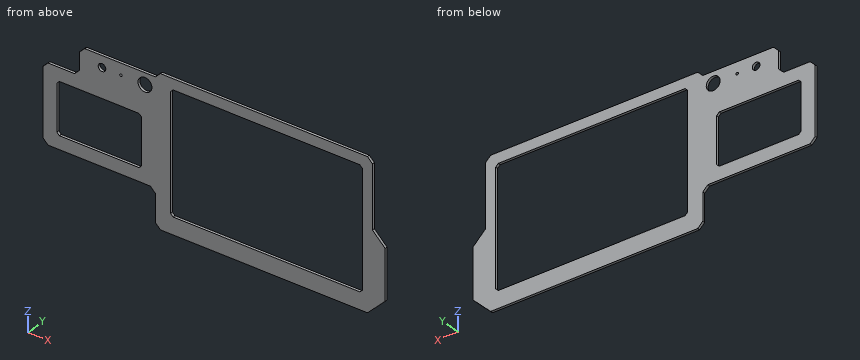
Autodesk Inventor part; units mm, degrees
ref_plane "YZ Plane" through (0, 0, 0) normal (1, 0, 0) x (0, 1, 0)
ref_plane "XZ Plane" through (0, 0, 0) normal (0, 1, 0) x (-1, 0, 0)
ref_plane "XY Plane" through (0, 0, 0) normal (0, 0, 1) x (1, 0, 0)
sketch "Sketch1" plane through (0, 0, 0) normal (0, 1, 0) x (-1, 0, 0)
  line L0 (0, -41) -> (-67, -41)
  line L1 (-67, -41) -> (-67, 0)
  line L2 (-67, 0) -> (0, 0)
  line L3 (0, 0) -> (0, -41)
  line L4 (-90, -68) -> (-242, -68)
  line L5 (-242, -68) -> (-242, 28)
  line L6 (-242, 28) -> (-90, 28)
  line L7 (-90, 28) -> (-90, -68)
  line L8 (11, -47.5) -> (11, 6.5)
  line L9 (7, 10.5) -> (-74, 10.5)
  line L10 (-78, 14.5) -> (-78, 32.5)
  line L11 (-82, 36.5) -> (-246, 36.5)
  line L12 (-250, 32.5) -> (-250, -77.5)
  line L13 (-246, -81.5) -> (-82, -81.5)
  line L14 (-78, -77.5) -> (-78, -55.5)
  line L15 (-74, -51.5) -> (7, -51.5)
  line L16 (11, -47.5) -> (7, -51.5)
  line L17 (-74, -51.5) -> (-78, -55.5)
  line L18 (-78, -77.5) -> (-82, -81.5)
  line L19 (-246, -81.5) -> (-250, -77.5)
  line L20 (-250, 32.5) -> (-246, 36.5)
  line L21 (-82, 36.5) -> (-78, 32.5)
  line L22 (-78, 14.5) -> (-74, 10.5)
  line L23 (7, 10.5) -> (11, 6.5)
  line L24 (6, -46.5) -> (-73, -46.5) construction
  line L25 (-73, -46.5) -> (-73, 5.5) construction
  line L26 (-73, 5.5) -> (6, 5.5) construction
  line L27 (6, 5.5) -> (6, -46.5) construction
  line L28 (-83, -76.5) -> (-245, -76.5) construction
  line L29 (-245, -76.5) -> (-245, 31.5) construction
  line L30 (-245, 31.5) -> (-83, 31.5) construction
  line L31 (-83, 31.5) -> (-83, -76.5) construction
  point P0 (11, 10.5)
  point P1 (-78, 10.5)
  point P2 (-78, 36.5)
  point P3 (-250, 36.5)
  point P4 (-250, -81.5)
  point P5 (-78, -81.5)
  point P6 (-78, -51.5)
  point P7 (11, -51.5)
  point P8 (-33.5, -46.5)
  point P9 (-33.5, -41)
  point P10 (6, -20.5)
  point P11 (0, -20.5)
  point P12 (-83, -22.5)
  point P13 (-90, -20)
  point P14 (-164, -76.5)
  point P15 (-166, -68)
  dimension "d0" = 67
  dimension "d1" = 41
  dimension "d2" = 152
  dimension "d3" = 96
  dimension "d4" = 4
  dimension "d5" = 4
  dimension "d6" = 4
  dimension "d7" = 4
  dimension "d8" = 4
  dimension "d9" = 4
  dimension "d10" = 4
  dimension "d11" = 4
  dimension "d12" = 4
  dimension "d13" = 4
  dimension "d14" = 4
  dimension "d15" = 4
  dimension "d16" = 4
  dimension "d17" = 4
  dimension "d18" = 4
  dimension "d19" = 4
  dimension "d20" = 79
  dimension "d21" = 52
  dimension "d22" = 162
  dimension "d23" = 108
  dimension "d24" = 10
  dimension "d25" = 26
  dimension "d26" = 5
  dimension "d27" = 5
  dimension "d28" = 5
  dimension "d29" = 5
  dimension "d30" = 5
  dimension "d31" = 5
  dimension "d32" = 5
  dimension "d48" = 8.5
  dimension "d49" = 7
extrude "Extrusion1" add sketch "Sketch1" along normal blind 2
sketch "Sketch2" plane through (0, 2, 0) normal (0, 1, 0) x (1, 0, 0)
  line L0 (250, -32.5) -> (250, 77.5)
  line L1 (78, 55.5) -> (74, 51.5)
  line L2 (74, 51.5) -> (-7, 51.5)
  line L3 (250, 77.5) -> (260, 67.5)
  line L4 (260, 67.5) -> (260, 27.5)
  line L5 (260, 27.5) -> (250, 17.5)
  line L6 (250, 77.5) -> (250, 17.5)
  dimension "d35" = 10
  dimension "d36" = 40
extrude "Extrusion2" add sketch "Sketch2" against normal blind 2
sketch "Sketch3" plane through (0, 2, 0) normal (0, 1, 0) x (1, 0, 0)
  line L0 (-7, -10.5) -> (74, -10.5)
  line L1 (74, -10.5) -> (78, -14.5)
  line L2 (78, -14.5) -> (78, -32.5)
  line L3 (78, 55.5) -> (74, 51.5)
  line L4 (74, 51.5) -> (-7, 51.5)
  line L5 (78, -32.5) -> (22, -32.5)
  line L6 (18, -28.5) -> (18, -14.5)
  line L7 (18, -14.5) -> (14, -10.5)
  line L8 (18, -28.5) -> (22, -32.5)
  line L9 (14, -10.5) -> (74, -10.5)
  line L10 (74, -10.5) -> (78, -14.5)
  line L11 (78, -14.5) -> (78, -32.5)
  point P0 (18, -32.5)
  dimension "d39" = 4
  dimension "d40" = 4
  dimension "d41" = 4
  dimension "d42" = 60
extrude "Extrusion3" add sketch "Sketch3" against normal blind 2
chamfer "Chamfer1" distance 2 angle 45 8 edges at (0, 1, -41) (67, 1, -41) (90, 1, -68) (90, 1, 28) (0, 1, 0) (67, 1, 0) (242, 1, 28) (242, 1, -68)
sketch "Sketch4" plane through (0, 2, 0) normal (0, 1, 0) x (1, 0, 0)
  line L0 (18, -14.5) -> (18, -28.5)
  line L1 (22, -32.5) -> (78, -32.5)
  circle A0 centre (69.75, -23.4) radius 5.5
  circle A1 centre (50.75, -23.4) radius 1
  circle A2 centre (35.75, -23.4) radius 3
  point P0 (0, 0)
  dimension "d50" = 11
  dimension "d51" = 2
  dimension "d52" = 6
  dimension "d53" = 19
  dimension "d54" = 15
  dimension "d55" = 9.1
  dimension "d56" = 51.75
extrude "Extrusion4" cut sketch "Sketch4" against normal through all
equation "\"d26\" = 0.5 * d24"
equation "\"d27\" = d26"
equation "\"d28\" = d27"
equation "\"d29\" = d28"
equation "\"d30\" = d26"
equation "\"d31\" = d30"
equation "\"d32\" = d30"
properties part number "front_panel_frame" material "ABS Plastic"
Verification items for the finished model (mm, model axes). Coordinates: 2 decimals unless noted, no trailing zeros. Loops run counter-clockwise (first coordinate to the right, second up) from the corner with the lowest first, then second, coordinate; pieces in that order, holes last. Notation, with made-up numbers: (36, 44) -> (85, 44) arc R11 cw to (85, 56) -> close; hole circle Ø1 at (48.5, 27.5). An arc over 180 degrees is marked (long way). Answer as a JSON object with one key per item and string values. Group by question number.
Item 1: Sectioned sample at B-B on x = 211. Record the boundary of the cut face in (y, z).
Item 2: Scan lines: probe 1 along Z at (x, y) = (50.75, 0.85); probe 2 along Z at (x, y) = (35.75, 0.65); probe 3 along X at (y, z) = (0.25, -17). Record each from-to range of solid material in increasing order.
Item 3: Depth check by flat-ended pin: pin 1 (1 mm diameter, centred on y = 0.5, z = 22.5, fed in from -X); pin 2 (2.5 mm diameter, centred on x = 50.75, z = 23.4, fed in from -Y); pin 3 (1 mm diameter, centred on x = 44.5, y = 1, fed in from +Z); pin 4 (1 mm diameter, centred on x = 19.5, y = 1, fed in from +Z). Enter the tip coordinate at first touch or a pass-through.
Item 4: Sectioned sample at C-C on x = 69.75. Record the boundary of the cut face in (y, z).
Item 5: Sectioned sample at D-D on y = 1.5. State how many separate pieces and enclosed holes the cut face has, plus the area to 3 significant figures.
Item 6: Sectioned sample at A-A on x = 35.75. Record the boundary of the cut face in (y, z).
Evaluation:
{
 "1": {"outline": "(0, -81.5) -> (2, -81.5) -> (2, -68) -> (0, -68) -> close; (0, 28) -> (2, 28) -> (2, 36.5) -> (0, 36.5) -> close"},
 "2": {"probe 1": "z = -51.5 to -41, 0 to 22.4, 24.4 to 32.5", "probe 2": "z = -51.5 to -41, 0 to 20.4, 26.4 to 32.5", "probe 3": "x = -11 to 0, 67 to 90, 242 to 250"},
 "3": {"pin 1": "stops at x = 18", "pin 2": "stops at y = 0", "pin 3": "stops at z = 32.5", "pin 4": "stops at z = 30.5"},
 "4": {"outline": "(0, -51.5) -> (2, -51.5) -> (2, 17.9) -> (0, 17.9) -> close; (0, 28.9) -> (2, 28.9) -> (2, 32.5) -> (0, 32.5) -> close"},
 "5": {"separate pieces": "1", "enclosed holes": "5", "area": "10,100 mm²"},
 "6": {"outline": "(0, -51.5) -> (2, -51.5) -> (2, -41) -> (0, -41) -> close; (0, 0) -> (2, 0) -> (2, 20.4) -> (0, 20.4) -> close; (0, 26.4) -> (2, 26.4) -> (2, 32.5) -> (0, 32.5) -> close"}
}
